```python
from build123d import *

# Parameters (mm, degrees)
SKETCH1_W                   = 90
SKETCH1_H                   = 90
SKETCH1_W_2                 = 80
SKETCH1_H_2                 = 80
BOSS_EXTRUDE1_DEPTH         = 10
SKETCH2_R                   = 3
BOSS_EXTRUDE2_DEPTH         = 20.5
BOSS_EXTRUDE3_DEPTH         = 5
BOSS_EXTRUDE3_DEPTH_BACK    = 5
BOSS_EXTRUDE4_START         = 15
SKETCH4_R                   = 3
BOSS_EXTRUDE4_DEPTH         = 15
BOSS_EXTRUDE5_DEPTH         = 10
BOSS_EXTRUDE6_DEPTH         = 4
SKETCH8_R                   = 1.5
BOSS_EXTRUDE7_DEPTH         = 5
BOSS_EXTRUDE7_TAPER         = 8
SKETCH9_R                   = 1.5
POST_FOR_RUBBER_BANDS_DEPTH = 1
MIRROR3_COPY_1_SKETCH_R     = 1.5
MIRROR3_COPY_1_DEPTH        = 5
MIRROR3_COPY_1_TAPER        = 8
MIRROR3_COPY_2_SKETCH_R     = 1.5
MIRROR3_COPY_2_DEPTH        = 1
SKETCH12_R                  = 0.889
BOSS_EXTRUDE10_DEPTH        = 10
CUT_EXTRUDE1_REACH          = 144.391
SKETCH13_R                  = 2


with BuildPart() as part:
    # Sketch1 → Boss-Extrude1 (new body)
    with BuildSketch(Plane(origin=(0, 0, 0), x_dir=(1, 0, 0), z_dir=(0, 1, 0))):
        Rectangle(SKETCH1_W, SKETCH1_H)
        Rectangle(SKETCH1_W_2, SKETCH1_H_2, mode=Mode.SUBTRACT)
    extrude(amount=BOSS_EXTRUDE1_DEPTH)

    # Sketch2 → Boss-Extrude2 (add)
    with BuildSketch(Plane(origin=(45, 0, 0), x_dir=(0, 0, -1), z_dir=(1, 0, 0))):
        with Locations(Location((0, 5, 0), (0, 0, 180))):
            Circle(SKETCH2_R)
    extrude(amount=BOSS_EXTRUDE2_DEPTH)

    # Sketch3 → Boss-Extrude3 (add, two sides: drawn at the far end of the back side and taken through both)
    with BuildSketch(Plane.XY.offset(-BOSS_EXTRUDE3_DEPTH_BACK)):
        Polygon((-40, 10), (-45, 10), (-5.084464777, 50), (5.084464777, 50), (45, 10), (40, 10), (5.07390668, 45), (-5.07390668, 45), align=None)
    extrude(amount=BOSS_EXTRUDE3_DEPTH + BOSS_EXTRUDE3_DEPTH_BACK)

    # Sketch4 → Boss-Extrude4 (add)
    with BuildSketch(Plane.ZY.offset(45).offset(BOSS_EXTRUDE4_START)):
        with Locations((0, 5)):
            Circle(SKETCH4_R)
    extrude(amount=-BOSS_EXTRUDE4_DEPTH)

    # Sketch5 → Boss-Extrude5 (add)
    with BuildSketch(Plane(origin=(0, 0, 0), x_dir=(1, 0, 0), z_dir=(0, 1, 0))):
        with BuildLine():
            Line((-40, -36.460175656), (-40, -40))
            Line((-40, -40), (-36.460175656, -40))
            Line((-36.460175656, -40), (-21.10179716, -23.0494394))
            ThreePointArc((-21.10179716, -23.0494394), (-31.25, 0), (-21.10179716, 23.0494394))
            Line((-21.10179716, 23.0494394), (-36.460175656, 40))
            Line((-36.460175656, 40), (-40, 40))
            Line((-40, 40), (-40, 36.460175656))
            Line((-40, 36.460175656), (-27.916615548, 23.124123255))
            ThreePointArc((-27.916615548, 23.124123255), (-36.25, 0), (-27.916615548, -23.124123255))
            Line((-27.916615548, -23.124123255), (-40, -36.460175656))
        make_face()
    boss_extrude5 = extrude(amount=BOSS_EXTRUDE5_DEPTH)

    # Mirror1: Boss-Extrude5 across plane
    add(boss_extrude5.mirror(Plane(origin=(0, 0, 0), x_dir=(0, 0, 1), z_dir=(1, 0, 0))))

    # Sketch6 → Boss-Extrude6 (add)
    with BuildSketch(Plane(origin=(0, 0, 0), x_dir=(1, 0, 0), z_dir=(0, 1, 0))):
        with BuildLine():
            ThreePointArc((-21.10179716, 23.0494394), (-22.883440442, 21.281697619), (-24.517477668, 19.376681574))
            ThreePointArc((-24.517477668, 19.376681574), (0, 8.693728204), (24.517477668, 19.376681574))
            ThreePointArc((24.517477668, 19.376681574), (22.883440442, 21.281697619), (21.10179716, 23.0494394))
            ThreePointArc((21.10179716, 23.0494394), (0, 13.693728204), (-21.10179716, 23.0494394))
        make_face()
        with BuildLine():
            ThreePointArc((-24.517477668, -19.376681574), (0, -8.693728204), (24.517477668, -19.376681574))
            ThreePointArc((24.517477668, -19.376681574), (22.883440442, -21.281697619), (21.10179716, -23.0494394))
            ThreePointArc((21.10179716, -23.0494394), (12.223024974, -16.450534785), (1.499479621, -13.733235994))
            ThreePointArc((1.499479621, -13.733235994), (0, -15.193728204), (-1.499479621, -13.733235994))
            ThreePointArc((-1.499479621, -13.733235994), (-12.223024974, -16.450534785), (-21.10179716, -23.0494394))
            ThreePointArc((-21.10179716, -23.0494394), (-22.883440442, -21.281697619), (-24.517477668, -19.376681574))
        make_face()
    extrude(amount=BOSS_EXTRUDE6_DEPTH)

    # Sketch8 → Boss-Extrude7 (add)
    with BuildSketch(Plane(origin=(0, 10, 0), x_dir=(1, 0, 0), z_dir=(0, 1, 0))):
        with Locations((-26.75, 20.224123255)):
            Circle(SKETCH8_R)
    boss_extrude7 = extrude(amount=BOSS_EXTRUDE7_DEPTH, taper=BOSS_EXTRUDE7_TAPER)

    # Sketch9 → Post for rubber bands (add)
    with BuildSketch(Plane(origin=(0, 15, 0), x_dir=(1, 0, 0), z_dir=(0, 1, 0))):
        with Locations(Location((-26.75, 20.224123255, 0), (0, 0, 270))):
            Circle(SKETCH9_R)
    post_for_rubber_bands = extrude(amount=POST_FOR_RUBBER_BANDS_DEPTH)

    # Mirror2: Boss-Extrude7, Post for rubber bands across plane
    add(boss_extrude7.mirror(Plane(origin=(0, 0, 0), x_dir=(0, 0, 1), z_dir=(1, 0, 0))))
    add(post_for_rubber_bands.mirror(Plane(origin=(0, 0, 0), x_dir=(0, 0, 1), z_dir=(1, 0, 0))))

    # Mirror3: Boss-Extrude7, Post for rubber bands across plane
    add(boss_extrude7.mirror(Plane.XY))
    add(post_for_rubber_bands.mirror(Plane.XY))

    # Mirror3 copy 1 sketch → Mirror3 copy 1 (add)
    with BuildSketch(Plane(origin=(0, 10, 0), x_dir=(-1, 0, 0), z_dir=(0, 1, 0))):
        with Locations((-26.75, 20.224123255)):
            Circle(MIRROR3_COPY_1_SKETCH_R)
    extrude(amount=MIRROR3_COPY_1_DEPTH, taper=MIRROR3_COPY_1_TAPER)

    # Mirror3 copy 2 sketch → Mirror3 copy 2 (add)
    with BuildSketch(Plane(origin=(0, 15, 0), x_dir=(-1, 0, 0), z_dir=(0, 1, 0))):
        with Locations(Location((-26.75, 20.224123255, 0), (0, 0, 270))):
            Circle(MIRROR3_COPY_2_SKETCH_R)
    extrude(amount=MIRROR3_COPY_2_DEPTH)

    # Sketch12 → Boss-Extrude10 (add)
    with BuildSketch(Plane(origin=(0, 41, 0), x_dir=(-1, 0, 0), z_dir=(0, -1, 0))):
        with Locations((-10.5, 0)):
            Circle(SKETCH12_R)
        with Locations(Location((10.5, 0, 0), (0, 0, 180))):
            Circle(SKETCH12_R)
    extrude(amount=BOSS_EXTRUDE10_DEPTH)

    # Sketch13 → Cut-Extrude1 (cut, up to next)
    with BuildSketch(Plane.ZY.offset(60), mode=Mode.PRIVATE) as cut_extrude1_sk1:
        with Locations((0, 5)):
            Circle(SKETCH13_R)
    cut_extrude1_tool1 = extrude(cut_extrude1_sk1.sketch, amount=-CUT_EXTRUDE1_REACH, mode=Mode.PRIVATE) & part.part
    add(cut_extrude1_tool1.solids().sort_by_distance((-60, 5, 0))[0], mode=Mode.SUBTRACT)


solid = part.part
```
Geometry: final body of the model. Coordinates: model frame, mm. A direction names the side the tool comes from. Round coordinates to 2 decimals unless told otherwise and drop trailing zeros. Write each loop counter-clockwise with the first axis right and the second up, starting at its lowest first coordinate (ties: lowest second). Pieces come first, ordered by that corner, then holes. Notation, with made-up numbers: M 12,27.25 L 49,27.25 A22 cw 49,55.25 Z; hole C -4.75,10.5 d4. An arc over 180 degrees is marked long. Answer in a Markdown table with one row per item. Add a question column.
(1) Contact query for flat-ended pins moving along their axis: pin 1 (3.5 mm diameter, centred on y = 5, z = 0, fed in from -X); pin 2 (12 mm diameter, centred on y = 20.5, z = -24.5, fed in from -X); pin 3 (3.5 mm diameter, centred on x = -26.5, z = 20.5, fed in from +Y); pin 4 (6 mm diameter, centred on y = 19, z = 23.5, fed in from -X). Output: stop coordinate, or through.
(2) Reachability of faces 4 (the face through (27.893, 12.535, 20.274)), 5 (the face through (0, 4, -13)), 6 (the face through (28.673, 4.93, -31.406)) from +Z, -Z, +X, -X, +Y, -Y: full face, straight path, thin tool, end or side. Return the list, or none.
(3) Draft query along Z for faces 1 (the face through (-1, 5, -45)), 2 (the face through (0.032, 1.972, 15.193)), 3 (the face through (0, 50, 0)). Return one class per face: pulls with the +Z half, pulls with the -Z half, needs draft (parallel to the pull), parting line crosses it, or undercut.
(4) Cut plane B-B, the plane y = 21. Return the cut outline in (x, z), then the cut area to 4 significant figures.
(5) Cut plane D-D, the plane y = 35. Return the cut outline in (x, z).
(6) Cut plane C-C, the plane z = 34.5. Return the cut outline in (x, y).
(7) Cut plane A-A, the plane x = 0. Return the cut outline in (y, z).
(8) Ray query, L1, parallel to Y at x = -50, z = 0; L2, parallel to X at y = 8.5, z = 4; L3, parallel to X at y = 4, z = 3.5. Return the intervals inside material, ascending.
Established:
| question | item | result |
|---|---|---|
| 1 | pin 1 | x = -36.25 |
| 1 | pin 2 | x = -28.22 |
| 1 | pin 3 | y = 16 |
| 1 | pin 4 | through |
| 2 | face 4 | none |
| 2 | face 5 | +Y |
| 2 | face 6 | +Y, -Y |
| 3 | face 1 | pulls with the -Z half |
| 3 | face 2 | undercut |
| 3 | face 3 | needs draft |
| 4 | outline | M -34.02,-5 L -29.02,-5 L -29.02,5 L -34.02,5 Z; M 29.02,-5 L 34.02,-5 L 34.02,5 L 29.02,5 Z |
| 4 | area | 100.0 mm² |
| 5 | outline | M -20.05,-5 L -15.05,-5 L -15.05,5 L -20.05,5 Z; C -10.5,0 d1.78; C 10.5,0 d1.78; M 15.05,-5 L 20.05,-5 L 20.05,5 L 15.05,5 Z |
| 6 | outline | M -45,0 L -40,0 L -40,10 L -45,10 Z; M -38.22,0 L -31.48,0 L -31.48,10 L -38.22,10 Z; M 31.48,0 L 38.22,0 L 38.22,10 L 31.48,10 Z; M 40,0 L 45,0 L 45,10 L 40,10 Z |
| 7 | outline | M 0,-45 L 10,-45 L 10,-40 L 0,-40 Z; M 0,-13.69 L 4,-13.69 L 4,-8.69 L 0,-8.69 Z; M 0,8.69 L 4,8.69 L 4,15.19 L 0,15.19 Z; M 0,40 L 10,40 L 10,45 L 0,45 Z; M 45,-5 L 50,-5 L 50,5 L 45,5 Z |
| 8 | L1 | 2 to 3, 7 to 8 |
| 8 | L2 | -45 to -40, -36.03 to -30.99, 30.99 to 36.03, 40 to 45 |
| 8 | L3 | -45 to -40, -36.08 to -31.05, 31.05 to 36.08, 40 to 45 |
